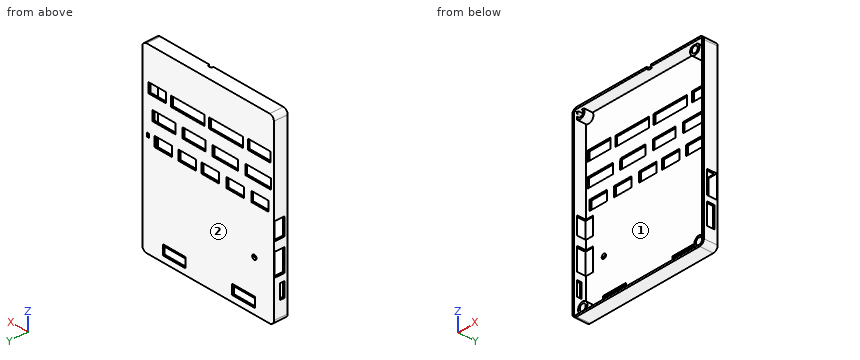
from build123d import *

# Parameters (mm, degrees)
SKETCH3_W            = 62.732633811
SKETCH3_H            = 79.574938689
SKETCH3_W_2          = 61.132633811
SKETCH3_H_2          = 77.974938689
BOSS_EXTRUDE8_DEPTH  = 6
SKETCH2_R            = 2.2
SKETCH2_R_2          = 1.409397898
BOSS_EXTRUDE9_DEPTH  = 4.6
SKETCH4_W            = 61.132633811
SKETCH4_H            = 77.974938689
BOSS_EXTRUDE11_DEPTH = 0.8
CUT_EXTRUDE2_DEPTH   = 4
SKETCH8_W            = 6.35
SKETCH8_H            = 1.7
SKETCH8_W_2          = 9.791634441
SKETCH8_H_2          = 4.4
SKETCH8_W_3          = 7.621
CUT_EXTRUDE3_DEPTH   = 1
SKETCH10_R           = 1
CUT_EXTRUDE4_DEPTH   = 10
SKETCH11_W           = 62.732633811
SKETCH11_H           = 0.53
CUT_EXTRUDE5_DEPTH   = 10
SKETCH12_W           = 61.132633811
SKETCH12_H           = 0.529997491
BOSS_EXTRUDE12_DEPTH = 6
BOSS_EXTRUDE14_DEPTH = 6
SKETCH16_W           = 0.807943928
SKETCH16_H           = 79.044938689
CUT_EXTRUDE6_DEPTH   = 10
CUT_EXTRUDE7_DEPTH   = 10
SKETCH20_W           = 9.7916
SKETCH20_H           = 4.3
SKETCH20_W_2         = 7.621
CUT_EXTRUDE9_DEPTH   = 4
FILLET1_R            = 2


with BuildPart() as part:
    # Sketch3 → Boss-Extrude8 (new body)
    with BuildSketch(Plane(origin=(0, 0, 0), x_dir=(1, 0, 0), z_dir=(0, 1, 0))):
        with Locations((27.16866126, -36.269344827)):
            Rectangle(SKETCH3_W, SKETCH3_H)
        with Locations((27.16866126, -36.269344827)):
            Rectangle(SKETCH3_W_2, SKETCH3_H_2, mode=Mode.SUBTRACT)
    extrude(amount=-BOSS_EXTRUDE8_DEPTH)

    # Sketch2 → Boss-Extrude9 (add)
    with BuildSketch(Plane(origin=(0, 0, 0), x_dir=(1, 0, 0), z_dir=(0, 1, 0))):
        Circle(SKETCH2_R)
        Circle(SKETCH2_R_2, mode=Mode.SUBTRACT)
        with Locations((54.706786111, 0.127852524)):
            Circle(SKETCH2_R)
        with Locations((54.706786111, 0.127852524)):
            Circle(SKETCH2_R_2, mode=Mode.SUBTRACT)
        with Locations((52.730413392, -72.978026956)):
            Circle(SKETCH2_R)
        with Locations((52.730413392, -72.978026956)):
            Circle(SKETCH2_R_2, mode=Mode.SUBTRACT)
        with Locations((-1.28124336, -73.51791918)):
            Circle(SKETCH2_R)
        with Locations((-1.28124336, -73.51791918)):
            Circle(SKETCH2_R_2, mode=Mode.SUBTRACT)
    extrude(amount=-BOSS_EXTRUDE9_DEPTH)

    # Sketch4 → Boss-Extrude11 (add)
    with BuildSketch(Plane(origin=(0, 0, 0), x_dir=(1, 0, 0), z_dir=(0, 1, 0))):
        with Locations((27.16866126, -36.269344827)):
            Rectangle(SKETCH4_W, SKETCH4_H)
    extrude(amount=-BOSS_EXTRUDE11_DEPTH)

    # Sketch7 → Cut-Extrude2 (cut)
    with BuildSketch(Plane(origin=(58.534978165, 0, 0), x_dir=(0, 0, -1), z_dir=(1, 0, 0))):
        Polygon((-3.898875483, -4.6), (-3.898875483, -2.1), (-3.898875483, -1.5), (-3.898875483, -1.4), (-13.125875483, -1.4), (-13.125875483, -1.5), (-13.125875483, -2.1), (-13.125875483, -4.6), align=None)
        Polygon((-15.492875483, -4.6), (-15.492875483, -0.6), (-15.492875483, -0.33), (-25.398875483, -0.33), (-25.398875483, -0.6), (-25.398875483, -4.6), align=None)
    extrude(amount=-CUT_EXTRUDE2_DEPTH, mode=Mode.SUBTRACT)

    # Sketch8 → Cut-Extrude3 (cut)
    with BuildSketch(Plane.ZY.offset(4.197655646)):
        with Locations((8.256875483, -3.75)):
            Rectangle(SKETCH8_W, SKETCH8_H)
        with Locations((19.363058263, -2.4)):
            Rectangle(SKETCH8_W_2, SKETCH8_H_2)
        with Locations((32.006375483, -2.4)):
            Rectangle(SKETCH8_W_3, SKETCH8_H_2)
    extrude(amount=-CUT_EXTRUDE3_DEPTH, mode=Mode.SUBTRACT)

    # Sketch10 → Cut-Extrude4 (cut)
    with BuildSketch(Plane(origin=(0, 0, 0), x_dir=(1, 0, 0), z_dir=(0, 1, 0))):
        with Locations((5.825978165, -18.159875483)):
            Circle(SKETCH10_R)
        Polygon((44.485978165, -38.144875483), (44.485978165, -41.994875483), (44.485978165, -42.394875483), (52.725978165, -42.394875483), (52.725978165, -38.144875483), (52.365978165, -38.144875483), align=None)
        Polygon((33.166978165, -38.144875483), (33.166978165, -41.994875483), (33.166978165, -42.394875483), (41.426978165, -42.394875483), (41.426978165, -38.144875483), (41.046978165, -38.144875483), align=None)
        Polygon((22.401978165, -41.994875483), (22.401978165, -38.274875483), (30.291978165, -38.274875483), (30.651978165, -38.274875483), (30.651978165, -42.524875483), (22.401978165, -42.524875483), align=None)
        Polygon((10.606978165, -38.144875483), (10.606978165, -41.994875483), (10.606978165, -42.394875483), (18.816978165, -42.394875483), (18.816978165, -38.144875483), (18.456978165, -38.144875483), align=None)
        Polygon((-0.950021835, -41.994875483), (-0.950021835, -38.274875483), (6.899978165, -38.274875483), (7.269978165, -38.274875483), (7.269978165, -42.534875483), (-0.950021835, -42.534875483), align=None)
        Polygon((25.154978165, -47.115875483), (13.774978165, -47.115875483), (13.524978165, -47.115875483), (13.552673933, -51.415875483), (13.774978165, -51.415875483), (25.524978165, -51.415875483), (25.524978165, -47.115875483), align=None)
        Polygon((-1.756021835, -47.115875483), (9.663978165, -47.115875483), (10.023978165, -47.115875483), (10.023978165, -51.425875483), (-1.756021835, -51.425875483), (-1.976021835, -51.425875483), (-1.976021835, -47.115875483), align=None)
        Polygon((47.402978165, -57.067875483), (55.012978165, -57.067875483), (55.652978165, -57.067875483), (55.652978165, -61.317875483), (47.402978165, -61.317875483), (47.402978165, -60.917875483), align=None)
        Polygon((38.146978165, 0.382124517), (38.146978165, -3.385875483), (48.535978165, -3.385875483), (48.895978165, -3.385875483), (48.895978165, 0.872124517), (38.146978165, 0.872124517), align=None)
        Polygon((15.896978165, -3.385875483), (5.507978165, -3.385875483), (5.507978165, 0.382124517), (5.507978165, 0.872124517), (16.256978165, 0.872124517), (16.256978165, -3.385875483), align=None)
        Polygon((53.361978165, -47.415875483), (43.784978165, -47.415875483), (42.974978165, -47.415875483), (42.974978165, -51.665875483), (43.784978165, -51.665875483), (53.721978165, -51.665875483), (53.721978165, -47.415875483), align=None)
        Polygon((29.687978165, -47.415875483), (39.264978165, -47.415875483), (39.624978165, -47.415875483), (39.624978165, -51.675875483), (29.687978165, -51.675875483), (28.876408648, -51.675875483), (28.876408648, -47.415875483), align=None)
        Polygon((-1.793021835, -57.197875483), (-1.793021835, -60.917875483), (-1.793021835, -61.447875483), (8.896978165, -61.447875483), (8.896978165, -57.197875483), (8.706978165, -57.197875483), align=None)
        Polygon((29.275978165, -56.837875483), (29.275978165, -60.917875483), (29.275978165, -61.087875483), (45.073978165, -61.087875483), (45.073978165, -56.837875483), (44.753978165, -56.837875483), align=None)
        Polygon((11.239978165, -56.837875483), (11.239978165, -60.917875483), (11.239978165, -61.087875483), (27.039978165, -61.087875483), (27.039978165, -56.837875483), (26.719978165, -56.837875483), align=None)
        Polygon((56.285232814, -41.994875483), (55.509188938, -41.994875483), (55.509188938, -40.403875483), (56.385232814, -40.403875483), (56.385232814, -41.994875483), align=None)
    extrude(amount=-CUT_EXTRUDE4_DEPTH, mode=Mode.SUBTRACT)

    # Sketch11 → Cut-Extrude5 (cut)
    with BuildSketch(Plane(origin=(0, 0, 0), x_dir=(1, 0, 0), z_dir=(0, 1, 0))):
        with Locations((27.16866126, -75.791814172)):
            Rectangle(SKETCH11_W, SKETCH11_H)
    extrude(amount=-CUT_EXTRUDE5_DEPTH, mode=Mode.SUBTRACT)

    # Sketch12 → Boss-Extrude12 (add)
    with BuildSketch(Plane.XZ.offset(6)):
        with Locations((27.16866126, 74.991815427)):
            Rectangle(SKETCH12_W, SKETCH12_H)
    extrude(amount=-BOSS_EXTRUDE12_DEPTH)

    # Sketch15 → Boss-Extrude14 (add)
    with BuildSketch(Plane.XZ.offset(6)):
        Polygon((-3.397655646, 74.726816681), (-2.587655646, 74.726816681), (-2.587655646, -2.718124517), (-2.587655646, -3.518124517), (-3.397655646, -3.518124517), align=None)
    extrude(amount=-BOSS_EXTRUDE14_DEPTH)

    # Sketch16 → Cut-Extrude6 (cut)
    with BuildSketch(Plane.XZ.offset(6)):
        with Locations((-3.793683682, 36.004344827)):
            Rectangle(SKETCH16_W, SKETCH16_H)
    extrude(amount=-CUT_EXTRUDE6_DEPTH, mode=Mode.SUBTRACT)

    # Sketch17 → Cut-Extrude7 (cut)
    with BuildSketch(Plane.XY.offset(75.526814172)):
        with BuildLine():
            Line((31.534978165, -6), (33.534978165, -6))
            ThreePointArc((33.534978165, -6), (32.534978165, -5), (31.534978165, -6))
        make_face()
    extrude(amount=-CUT_EXTRUDE7_DEPTH, mode=Mode.SUBTRACT)

    # Sketch20 → Cut-Extrude9 (cut)
    with BuildSketch(Plane.ZY.offset(3.389711718)):
        Polygon((5.081875483, -4.6), (5.081875483, -2.9), (5.081875483, -2.75), (11.431875483, -2.75), (11.431875483, -2.9), (11.431875483, -4.6), align=None)
        with Locations((19.367675483, -2.45)):
            Rectangle(SKETCH20_W, SKETCH20_H)
        with Locations((32.002375483, -2.45)):
            Rectangle(SKETCH20_W_2, SKETCH20_H)
    extrude(amount=-CUT_EXTRUDE9_DEPTH, mode=Mode.SUBTRACT)

    # Fillet1
    fillet1_edges = [part.edges().sort_by_distance(p)[0] for p in [
        (58.534978165, -3, 75.526814172),
        (-3.389711718, -3, 75.526814172),
        (-3.389711718, -3, -3.518124517),
        (58.534978165, -3, -3.518124517),
    ]]
    fillet(fillet1_edges, radius=FILLET1_R)


solid = part.part
The listing builds one solid part. Answer for the finished solid, in the listing's coordinates (mm). Face numbers are marked on the shaded views. Give positions to 0.01 mm unless a question says otherwise; leave off trailing zeros. Write each loop counter-clockwise with the first axis right and the second up, starting at its lowest first coordinate (ties: lowest second). Pieces come first, ordered by that corner, then holes. Notation, with made-up numbers: (71, -37) -> (116, -37) arc R24 ccw to (116, -27) -> close; hole circle Ø2 at (34, 2.25). An arc over 180 degrees is marked (long way). Use a Markdown table: item, result.
(1) Section C-C, the plane z = 69 is taken. Determine the outline of the cut face in (x, y).
Return value:
| item | result |
|---|---|
| outline | (-3.39, -6) -> (-2.59, -6) -> (-2.59, -0.8) -> (57.73, -0.8) -> (57.73, -6) -> (58.53, -6) -> (58.53, 0) -> (-3.39, 0) -> close |
(2) Section A-A, the plane z = 34 is taken. Determine the outline of the cut face in (x, y).
Return value:
| item | result |
|---|---|
| outline | (-3.39, -6) -> (-2.59, -6) -> (-2.59, -4.6) -> (-3.39, -4.6) -> close; (-3.39, -0.3) -> (0.61, -0.3) -> (0.61, -0.8) -> (57.73, -0.8) -> (57.73, -6) -> (58.53, -6) -> (58.53, 0) -> (-3.39, 0) -> close |
(3) Find the intervals of material crossed by probe 1 along Z at (x, y) = (24, -0.75); probe 2 along Z at (x, y) = (43, -4.35); probe 3 along Z at (x, y) = (0, -2.5), in increasing order. Write a range as from..to.
Return value:
| item | result |
|---|---|
| probe 1 | -3.52..38.27, 42.52..47.12, 51.42..56.84, 61.09..75.53 |
| probe 2 | -3.52..-2.72, 74.73..75.53 |
| probe 3 | -3.52..-2.72, -2.2..-1.41, 1.41..2.2, 71.73..72.93, 74.11..75.53 |
(4) Determine the mould class of the marked faces 1 and 2 for opening direction X: released by +X, released by -X, zero draft, split by the parting line, or undercut.
Return value:
| item | result |
|---|---|
| face 1 | undercut |
| face 2 | zero draft |
(5) Flat-ended cylindrical pins translate along their axes: P1, Ø1.7, axis at x = 52.73, z = 72.98, coming from the -Y side; P2, Ø0.9, axis at x = 58.5, y = -2.5, coming from the +Z side. Find the tip coordinate at first contact, or state that the pin passes through.
Return value:
| item | result |
|---|---|
| P1 | y = -0.8 |
| P2 | z = 74.83 |
(6) Section B-B, the plane x = 4 is taken. Determine the outline of the cut face in (y, z).
Return value:
| item | result |
|---|---|
| outline | (-6, -3.52) -> (0, -3.52) -> (0, 38.27) -> (-0.8, 38.27) -> (-0.8, -2.72) -> (-6, -2.72) -> close; (-6, 74.73) -> (-0.8, 74.73) -> (-0.8, 61.45) -> (0, 61.45) -> (0, 75.53) -> (-6, 75.53) -> close; (-0.8, 42.53) -> (0, 42.53) -> (0, 47.12) -> (-0.8, 47.12) -> close; (-0.8, 51.43) -> (0, 51.43) -> (0, 57.2) -> (-0.8, 57.2) -> close |
